```python
from build123d import *

# Parameters (mm, degrees)
SKETCH1_W           = 190
SKETCH1_H           = 105
BOSS_EXTRUDE1_DEPTH = 140
CHAMFER1_SIZE       = 190.811366877
CHAMFER1_SIZE_2     = 10
SHELL1_T            = -3


with BuildPart() as part:
    # Sketch1 → Boss-Extrude1 (new body)
    with BuildSketch(Plane.XY):
        with Locations((-15.339943343, 4.194995279)):
            Rectangle(SKETCH1_W, SKETCH1_H)
    extrude(amount=BOSS_EXTRUDE1_DEPTH)

    # Chamfer1
    # the kernel refuses this chamfer: 190.811366877, 10 mm, written as the material it takes off along each edge
    with BuildSketch(Plane(origin=(-606.424352322, 56.694995279, 140), x_dir=(0, 0.00201302342238207, -0.9999979738662977), z_dir=(1, 0, 0)), Plane(origin=(575.744465637, -48.305004721, 140), x_dir=(0, -0.00201302342238207, -0.9999979738662977), z_dir=(-1, 0, 0))) as chamfer1_piece_1:
        Polygon((CHAMFER1_SIZE * 0.999997973868, -CHAMFER1_SIZE * 0.00201302342239), (-CHAMFER1_SIZE_2 * 0.00201302342238, -CHAMFER1_SIZE_2 * 0.999997973866), (0, 0), align=None)
    extrude(amount=1182.168817959, mode=Mode.SUBTRACT)
    with BuildSketch(Plane(origin=(79.660056657, 552.779404258, 140), x_dir=(0.0020130234223821055, 0, -0.9999979738662977), z_dir=(0, -1, 0)), Plane(origin=(-110.339943343, -544.389413701, 140), x_dir=(-0.0020130234223821055, 0, -0.9999979738662977), z_dir=(0, 1, 0))) as chamfer1_piece_2:
        Polygon((CHAMFER1_SIZE * 0.999997973868, -CHAMFER1_SIZE * 0.00201302342239), (-CHAMFER1_SIZE_2 * 0.00201302342238, -CHAMFER1_SIZE_2 * 0.999997973866), (0, 0), align=None)
    extrude(amount=1097.168817959, mode=Mode.SUBTRACT)

    # Shell1
    shell1_openings = [part.faces().sort_by_distance(p)[0] for p in [
        (-15.339943343, 4.194995279, 0),
    ]]
    offset(amount=SHELL1_T, openings=shell1_openings, kind=Kind.INTERSECTION)


solid = part.part
```
Here's how the part is built. I have some questions about the finished solid (model axes, mm). A direction names the side the tool comes from. Give positions to 0.01 mm unless a question says otherwise; leave off trailing zeros. Order: outer loops, then holes, each group sorted by start corner. A loop starts at its lowest first (then second) coordinate and runs counter-clockwise, first axis right, second up. Notation, with made-up numbers: M 80,67 L 126,67 A17 cw 126,99 Z; hole C 53,31.25 d2. An arc over 180 degrees is marked long. Use a Markdown table: item, result. Add a question column.
1. If we mould it in two halves opening along X, with no side actions, what happens to faces 1 (the flat face through (-43, -44, 0)), 2 (the flat face through (70.453, 4.851, 67.541)), 3 (the flat face through (73.38, 4.89, 69.02))? For each: +X half, -X half, draft (parallel to the pull), parting line (faces both ways), or undercut.
2. Suppose I cut it at A-A (x = -41). List the corners of the cut face in (y, z) for me (3 decimals), and give its area (3 significant figures).
3. I need wall thicknesses on probe 1 along Z at (x, y) = (51.5, -16); probe 2 along X at (y, z) = (1, 79); probe 3 along X at (y, z) = (39.5, 125). Which ranges of each line are inside material? Lowest first, please. Write a range as from..to.
4. Suppose I cut it at B-B (z = 30.5). List the corners of the cut face in (x, y) for me, and give its area (3 significant figures).
5. Suppose I cut it at C-C (y = -27). List the corners of the cut face in (x, z) for me, and give its area (3 significant figures).
6. For pin 1 Ø2 at (y, z) = (-32, 119.5) entering from -X; pin 2 Ø8 at (x, z) = (-12, 75.5) entering from -Y; pin 3 Ø3 at (x, z) = (53, 76) entering from +Y, each with a flat end and sliding along its axis, tell me the tip position at first contact or that it passes through.
7. On a 3-axis mill with a long thin cutter (end or side, diameter ignored), from which of +Z, -Z, +X, -X, +Y, -Y can I reach the whole of each face in a straight line? I mean faces 4 (the flat face through (-14.047, -42.025, 69.02)), 5 (the flat face through (-101.133, 3.539, 67.541)). Say none if no direction works.
8. Suppose I cut it at D-D (z = 9). List the corners of the cut face in (x, y) for me.
Results list:
| question | item | result |
|---|---|---|
| 1 | face 1 | draft |
| 1 | face 2 | undercut |
| 1 | face 3 | +X half |
| 2 | outline | M -45.642,0 L -42.638,0 L -35.458,137 L 43.848,137 L 51.028,0 L 54.032,0 L 46.695,140 L -38.305,140 Z |
| 2 | area | 1,080 mm² |
| 3 | probe 1 | z = 137..140 |
| 3 | probe 2 | x = -103.54..-100.53, 69.85..72.86 |
| 3 | probe 3 | x = -101.13..-98.12, 67.44..70.45 |
| 4 | outline | M -106.08,-44.04 L 75.4,-44.04 L 75.4,52.43 L -106.08,52.43 Z; hole M -103.07,-41.04 L 72.39,-41.04 L 72.39,49.43 L -103.07,49.43 Z |
| 4 | area | 1,630 mm² |
| 5 | outline | M -107.68,0 L -104.67,0 L -97.49,137 L 66.81,137 L 73.99,0 L 77,0 L 69.66,140 L -100.34,140 Z |
| 5 | area | 1,330 mm² |
| 6 | pin 1 | stops at x = -101.47 |
| 6 | pin 2 | stops at y = -41.89 |
| 6 | pin 3 | stops at y = 50.13 |
| 7 | face 4 | +Z, +X, -X, -Y |
| 7 | face 5 | -Z |
| 8 | outline | M -107.21,-45.17 L 76.53,-45.17 L 76.53,53.56 L -107.21,53.56 Z; hole M -104.2,-42.17 L 73.52,-42.17 L 73.52,50.56 L -104.2,50.56 Z |
